Work out the finished part from the listing and answer in its coordinate system (mm). Round coordinates to 2 decimals unless told otherwise and drop trailing zeros. Write each loop counter-clockwise with the first axis right and the second up, starting at its lowest first coordinate (ties: lowest second). Pieces come first, ordered by that corner, then holes. Notation, with made-up numbers: (59.25, 43) -> (77.25, 43) arc R11 ccw to (77.25, 55) -> close; hole circle Ø6 at (-20, 42). An arc over 180 degrees is marked (long way). One line per item, written item: value.
```python
from build123d import *

# Parameters (mm, degrees)
SZKIC1_W                    = 374
SZKIC1_H                    = 53
DODANIE_WYCI_GNI_CIE1_DEPTH = 1
SZKIC6_W                    = 31
SZKIC6_H                    = 2
WYTNIJ_WYCI_GNI_CIE1_DEPTH  = 2
SZKIC7_W                    = 374
SZKIC7_H                    = 53
SZKIC7_W_2                  = 373
SZKIC7_H_2                  = 52
WYTNIJ_WYCI_GNI_CIE2_DEPTH  = 10


with BuildPart() as part:
    # Szkic1 → Dodanie-wyciągnięcie1 (new body)
    with BuildSketch(Plane.XY):
        Rectangle(SZKIC1_W, SZKIC1_H)
    extrude(amount=DODANIE_WYCI_GNI_CIE1_DEPTH)

    # Szkic6 → Wytnij-wyciągnięcie1 (cut)
    with BuildSketch(Plane(origin=(0, 0, 0), x_dir=(-1, 0, 0), z_dir=(0, 0, -1))):
        with Locations((-166.5, -5.6)):
            Rectangle(SZKIC6_W, SZKIC6_H)
        with Locations((-129.5, -5.6)):
            Rectangle(SZKIC6_W, SZKIC6_H)
        with Locations((-92.5, -5.6)):
            Rectangle(SZKIC6_W, SZKIC6_H)
        with Locations((-18.5, -5.6)):
            Rectangle(SZKIC6_W, SZKIC6_H)
        with Locations((18.5, -5.6)):
            Rectangle(SZKIC6_W, SZKIC6_H)
        with Locations((55.5, -5.6)):
            Rectangle(SZKIC6_W, SZKIC6_H)
        with Locations((92.5, -5.6)):
            Rectangle(SZKIC6_W, SZKIC6_H)
        with Locations((129.5, -5.6)):
            Rectangle(SZKIC6_W, SZKIC6_H)
        with Locations((166.5, -5.6)):
            Rectangle(SZKIC6_W, SZKIC6_H)
        with Locations((-129.5, -24)):
            Rectangle(SZKIC6_W, SZKIC6_H)
        with Locations((-166.5, 24)):
            Rectangle(SZKIC6_W, SZKIC6_H)
        with Locations((-166.5, -24)):
            Rectangle(SZKIC6_W, SZKIC6_H)
        with Locations((-129.5, 24)):
            Rectangle(SZKIC6_W, SZKIC6_H)
        with Locations((-92.5, -24)):
            Rectangle(SZKIC6_W, SZKIC6_H)
        with Locations((-92.5, 24)):
            Rectangle(SZKIC6_W, SZKIC6_H)
        with Locations((-55.5, -24)):
            Rectangle(SZKIC6_W, SZKIC6_H)
        with Locations((-55.5, 24)):
            Rectangle(SZKIC6_W, SZKIC6_H)
        with Locations((-18.5, -24)):
            Rectangle(SZKIC6_W, SZKIC6_H)
        with Locations((-18.5, 24)):
            Rectangle(SZKIC6_W, SZKIC6_H)
        with Locations((18.5, -24)):
            Rectangle(SZKIC6_W, SZKIC6_H)
        with Locations((18.5, 24)):
            Rectangle(SZKIC6_W, SZKIC6_H)
        with Locations((55.5, -24)):
            Rectangle(SZKIC6_W, SZKIC6_H)
        with Locations((55.5, 24)):
            Rectangle(SZKIC6_W, SZKIC6_H)
        with Locations((92.5, -24)):
            Rectangle(SZKIC6_W, SZKIC6_H)
        with Locations((92.5, 24)):
            Rectangle(SZKIC6_W, SZKIC6_H)
        with Locations((129.5, -24)):
            Rectangle(SZKIC6_W, SZKIC6_H)
        with Locations((129.5, 24)):
            Rectangle(SZKIC6_W, SZKIC6_H)
        with Locations((166.5, -24)):
            Rectangle(SZKIC6_W, SZKIC6_H)
        with Locations((166.5, 24)):
            Rectangle(SZKIC6_W, SZKIC6_H)
        with Locations((-129.5, 5.6)):
            Rectangle(SZKIC6_W, SZKIC6_H)
        with Locations((-55.5, -5.6)):
            Rectangle(SZKIC6_W, SZKIC6_H)
        with Locations((-166.5, 5.6)):
            Rectangle(SZKIC6_W, SZKIC6_H)
        with Locations((-92.5, 5.6)):
            Rectangle(SZKIC6_W, SZKIC6_H)
        with Locations((-55.5, 5.6)):
            Rectangle(SZKIC6_W, SZKIC6_H)
        with Locations((-18.5, 5.6)):
            Rectangle(SZKIC6_W, SZKIC6_H)
        with Locations((18.5, 5.6)):
            Rectangle(SZKIC6_W, SZKIC6_H)
        with Locations((55.5, 5.6)):
            Rectangle(SZKIC6_W, SZKIC6_H)
        with Locations((92.5, 5.6)):
            Rectangle(SZKIC6_W, SZKIC6_H)
        with Locations((129.5, 5.6)):
            Rectangle(SZKIC6_W, SZKIC6_H)
        with Locations((166.5, 5.6)):
            Rectangle(SZKIC6_W, SZKIC6_H)
    extrude(amount=-WYTNIJ_WYCI_GNI_CIE1_DEPTH, mode=Mode.SUBTRACT)

    # Szkic7 → Wytnij-wyciągnięcie2 (cut)
    with BuildSketch(Plane(origin=(0, 0, 0), x_dir=(-1, 0, 0), z_dir=(0, 0, -1))):
        Rectangle(SZKIC7_W, SZKIC7_H)
        Rectangle(SZKIC7_W_2, SZKIC7_H_2, mode=Mode.SUBTRACT)
    extrude(amount=-WYTNIJ_WYCI_GNI_CIE2_DEPTH, mode=Mode.SUBTRACT)


solid = part.part
```
(1) Find section A-A on x = -130.5. Give the vertices of the cut face in (y, z).
Reported:
outline: (-26, 0) -> (-25, 0) -> (-25, 1) -> (-26, 1) -> close; (-23, 0) -> (-6.6, 0) -> (-6.6, 1) -> (-23, 1) -> close; (-4.6, 0) -> (4.6, 0) -> (4.6, 1) -> (-4.6, 1) -> close; (6.6, 0) -> (23, 0) -> (23, 1) -> (6.6, 1) -> close; (25, 0) -> (26, 0) -> (26, 1) -> (25, 1) -> close
(2) Find section B-B on z = 0.8. Give the number of separate pieces and of enclosed holes in the cut face, plus the area to 3 significant figures.
Reported:
separate pieces: 1
enclosed holes: 40
area: 16,900 mm2
(3) A flat-ended cylindrical pin translates along its axis: pin 1 Ø4 at (x, y) = (33, -5.5) entering from -Z. Find the tip coordinate at first contact, or state that the pin passes through.
Reported:
pin 1: stops at z = 0
(4) Consider probe 1 along Y at (x, z) = (152, 0.3). Determine where the line is inside the solid, lowest interval first.
Reported:
probe 1: y = -26 to -25, -23 to -6.6, -4.6 to 4.6, 6.6 to 23, 25 to 26
